CAD build for the part. Positions are in the model's coordinates, mm. Face numbers are marked on the shaded views. A direction names the side the tool comes from. Coordinates: 2 decimals unless noted, no trailing zeros. Order: outer loops, then holes, each group sorted by start corner. A loop starts at its lowest first (then second) coordinate and runs counter-clockwise, first axis right, second up. Notation, with made-up numbers: M -31.5,54.5 L 8.5,54.5 A30 ccw 8.5,87.5 Z; hole C 79.25,23.5 d2. An arc over 180 degrees is marked long. One line per item, written item: value.
from build123d import *

# Parameters (mm, degrees)
POCKET027_DEPTH       = 30
SKETCH032_R           = 2.2
POCKET028_DEPTH       = 284.142394
POLARPATTERN002_COUNT = 2
POLARPATTERN002_ANGLE = 240
SKETCH146_R           = 7.5
POCKET091_DEPTH       = 17.679838


with BuildPart() as part:
    # Sketch022 → Revolution001 (revolve)
    with BuildSketch(Plane.XY):
        Polygon((0, 26), (70.880385, 26), (72, 25.7), (84, 25.7), (84, 33), (72, 33), (72, 28), (2, 28), (1, 29), (0, 29), align=None)
    revolve(axis=Axis((0, 0, 0), (1, 0, 0)))

    # Sketch031 (on DatumPlane) → Pocket027 (cut)
    with BuildSketch(Plane(origin=(78, 0, 0), x_dir=(1, 0, 0), z_dir=(0, -1, 0))):
        Polygon((3.6, 2.078461), (0, 4.156922), (-3.6, 2.078461), (-3.6, -2.078461), (0, -4.156922), (3.6, -2.078461), align=None)
    pocket027 = extrude(amount=-POCKET027_DEPTH, mode=Mode.SUBTRACT)

    # Sketch032 (on DatumPlane) → Pocket028 (cut, through all)
    with BuildSketch(Plane(origin=(78, 0, 0), x_dir=(1, 0, 0), z_dir=(0, -1, 0))):
        Circle(SKETCH032_R)
    pocket028 = extrude(amount=-POCKET028_DEPTH, mode=Mode.SUBTRACT)

    # PolarPattern002: Pocket028, Pocket027 ×2 about axis
    polarpattern002_axis = Axis((0, 0, 0), (1, 0, 0))
    for i in range(1, POLARPATTERN002_COUNT):
        add(pocket028.rotate(polarpattern002_axis, i * POLARPATTERN002_ANGLE / (POLARPATTERN002_COUNT - 1)), mode=Mode.SUBTRACT)
        add(pocket027.rotate(polarpattern002_axis, i * POLARPATTERN002_ANGLE / (POLARPATTERN002_COUNT - 1)), mode=Mode.SUBTRACT)

    # Sketch146 (on DatumPlane) → Pocket091 (cut, through all)
    with BuildSketch(Plane(origin=(72, -13.7, 23.729096), x_dir=(1, 0, 0), z_dir=(0, 0.5, -0.866025))):
        with Locations((18, 0)):
            Circle(SKETCH146_R)
    extrude(amount=-POCKET091_DEPTH, mode=Mode.SUBTRACT)


with BuildPart() as part_1:
    # Body007 placement: moved
    add(part.part.moved(Location((110, 0, 834))))


solid = part_1.part
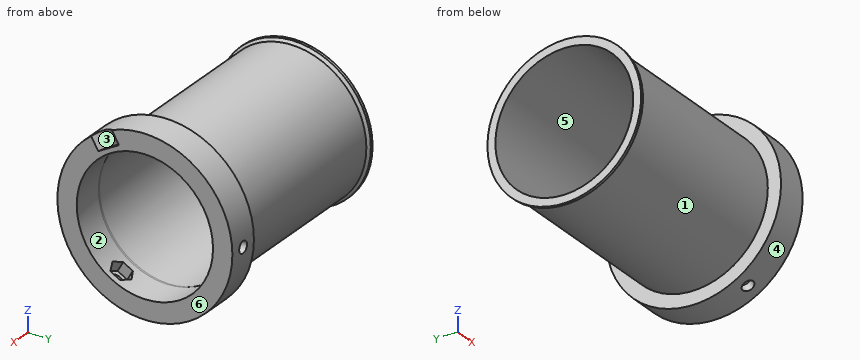
Q1. Slice it at C-C (x = 143.5). List the corners of the cut face in (y, z).
Recorded:
outline: C 0,834 d56; hole C 0,834 d52
Q2. Drill centre lines: line 1 along X through (y, z) = (31.05, 834); line 2 along Z through (x, y) = (189.5, 0); line 3 along Y through (x, z) = (166.5, 815.5). Where is each one in solid material? Low to high.
Recorded:
line 1: x = 182 to 185.8, 190.2 to 194
line 2: z = 801 to 808.3, 859.7 to 867
line 3: y = -21.02 to -18.27, 18.27 to 21.02
Q3. Mould opens along Y. For the marked faces 3, 4, 5 and 6 say: released by +Y, released by -Y, zero draft, split by the parting line, or undercut.
Recorded:
face 3: undercut
face 4: split by the parting line
face 5: undercut
face 6: zero draft
Q4. Pin check, flat tips, straight feed: pin 1 Ø3 at (x, z) = (136, 811.5) entering from +Y; pin 2 Ø1 at (x, y) = (125.5, -15) entering from -Z; pin 3 Ø4 at (x, z) = (188, 834) entering from +Y; pin 4 Ø8 at (x, z) = (187.5, 833) entering from -Y. Stop position of each tip, or through.
Recorded:
pin 1: stops at y = 18.52
pin 2: stops at z = 810.05
pin 3: stops at y = -25.62
pin 4: stops at y = -33
Q5. Which spindle directions (+Z, -Z, +X, -X, +Y, -Y) get a long thin tool onto all of the face, cutting with end or side? Do the marked faces 1 and 2. Say none if no direction does.
Recorded:
face 1: none
face 2: +X, -X
Q6. Slice it at A-A (z = 834). List the corners of the cut face in (x, y), plus the area to 3 significant figures.
Recorded:
outline: M 110,-29 L 111,-29 L 112,-28 L 182,-28 L 182,-33 L 194,-33 L 194,-25.7 L 182,-25.7 L 180.88,-26 L 110,-26 Z; M 110,26 L 180.88,26 L 182,25.7 L 184.4,25.7 L 184.4,30 L 185.8,30 L 185.8,33 L 182,33 L 182,28 L 112,28 L 111,29 L 110,29 Z; M 190.2,30 L 191.6,30 L 191.6,25.7 L 194,25.7 L 194,33 L 190.2,33 Z
area: 422 mm^2
Q7. Slice it at B-B (y = 0). List the corners of the cut face in (x, z), plus the area to 3 significant figures.
Recorded:
outline: M 110,805 L 111,805 L 112,806 L 182,806 L 182,801 L 194,801 L 194,808.3 L 182,808.3 L 180.88,808 L 110,808 Z; M 110,860 L 180.88,860 L 182,859.7 L 194,859.7 L 194,867 L 182,867 L 182,862 L 112,862 L 111,863 L 110,863 Z
area: 467 mm^2
